from build123d import *

# Parameters (mm, degrees)
F0_W     = 254
F0_H     = 254
F1_DEPTH = 254


with BuildPart() as f1:
    # F0 (on Front) → F1 (new body)
    with BuildSketch(Plane.XZ):
        with Locations((127, 127)):
            Rectangle(F0_W, F0_H)
        with BuildLine():
            ThreePointArc((50.8, 25.4), (29.193469, 37.44643), (28.081549, 62.159225))
            Line((28.081549, 62.159225), (104.281549, 214.559225))
            ThreePointArc((104.281549, 214.559225), (127, 228.6), (149.718451, 214.559225))
            Line((149.718451, 214.559225), (225.918451, 62.159225))
            ThreePointArc((225.918451, 62.159225), (224.806531, 37.44643), (203.2, 25.4))
            Line((203.2, 25.4), (50.8, 25.4))
        make_face(mode=Mode.SUBTRACT)
    extrude(amount=F1_DEPTH)


solid = f1.part
Here's how the part is built. I have some questions about the finished solid (model axes, mm). A direction names the side the tool comes from. Round coordinates to 2 decimals unless told otherwise and drop trailing zeros. Write each loop counter-clockwise with the first axis right and the second up, starting at its lowest first coordinate (ties: lowest second). Pieces come first, ordered by that corner, then holes.
1. Suppose I cut it at C-C (y = -165.5). List the corners of the cut face in (x, z) for me.
2. If we mould it in two halves opening along Z, with no side actions, what happens to faces 3 (the flat face through (125, -125, 0)), 4 (the cylindrical face through (126.606, -125.222, 228.597)), 5 (the flat face through (254, -125, 125)), 6 (the flat face through (125, -125, 254))? For each: released by +Z, released by -Z, zero draft, split by the parting line, or undercut.
3. I need wall thicknesses on L1, parallel to Z at x = 64, y = -228.5; L2, parallel to X at y = -39.5, z = 161; L3, parallel to X at y = -122.5, z = 41. Which ranges of each line are inside material? Lowest first, please.
4. Suppose I cut it at B-B (x = 131.5). List the corners of the cut face in (y, z) for me, and give its area (3 significant figures).
5. Suppose I cut it at A-A (z = 35.5). List the corners of the cut face in (x, y) for me.
6. For faces 1 (the cylindrical face through (29.386, -125.222, 37.14)), 2 (the flat face through (0, -125, 125)), which set-ups out of +Z, -Z, +X, -X, +Y, -Y let a thin tool reach every point of the face, with its end or its side?
Answer sheet:
1. outline: (0, 0) - (254, 0) - (254, 254) - (0, 254) - close; hole (28.08, 62.16) arc R25.4 ccw to (50.8, 25.4) - (203.2, 25.4) arc R25.4 ccw to (225.92, 62.16) - (149.72, 214.56) arc R25.4 ccw to (104.28, 214.56) - close
2. face 3: released by -Z
2. face 4: undercut
2. face 5: zero draft
2. face 6: released by +Z
3. L1: z = 0 to 25.4, 134 to 254
3. L2: x = 0 to 77.5, 176.5 to 254
3. L3: x = 0 to 27.37, 226.63 to 254
4. outline: (-254, 0) - (0, 0) - (0, 25.4) - (-254, 25.4) - close; (-254, 228.2) - (0, 228.2) - (0, 254) - (-254, 254) - close
4. area: 13,000 mm2
5. outline: (0, -254) - (30.53, -254) - (30.53, 0) - (0, 0) - close; (223.47, -254) - (254, -254) - (254, 0) - (223.47, 0) - close
6. face 1: +Y, -Y
6. face 2: +Z, -Z, -X, +Y, -Y
